Part model, mm, in its own coordinate system. Face numbers are marked on the shaded views. A direction names the side the tool comes from. Coordinates: 2 decimals unless noted, no trailing zeros. Loops run counter-clockwise (first coordinate to the right, second up) from the corner with the lowest first, then second, coordinate; pieces in that order, holes last. Notation, with made-up numbers: M -28.5,-9.75 L 15.5,-9.75 A28 ccw 15.5,29.25 Z; hole C -2.5,-7.75 d9. An arc over 180 degrees is marked long. Use a Markdown table: item, result. Add a question column.
1) Band-saw the part on C-C (z = 1.75). List the corners of the cut face in (x, y) (3 decimals).
2) Tool access for the marked faces 1, 2 and 3: list every direction of +Z, -Z, +X, -X, +Y, -Y with a clear straight run to the whole face (end or side of a thin tool).
3) Wall check: probe 1 along Y at (x, z) = (-0.5, 14.75) (3 decimals); probe 2 along Y at (x, z) = (9.75, 13.75) (3 decimals); probe 3 along Z at (x, y) = (1.75, -0.5). Give the ranges that are in metal, low to high. Write a range as from..to.
4) Pin check, flat tips, straight feed: pin 1 Ø1.5 at (x, y) = (-4, 7.5) entering from +Z; pin 2 Ø4 at (x, y) = (9.5, -2.5) entering from -Z. Stop position of each tip, or through.
5) Band-saw the part on A-A (x = 9.5). List the corners of the cut face in (y, z).
6) Band-saw the part on D-D (y = 5.5). List the corners of the cut face in (x, z).
7) Band-saw the part on B-B (y = -0.5). List the corners of the cut face in (x, z), plus the area to 3 significant figures.
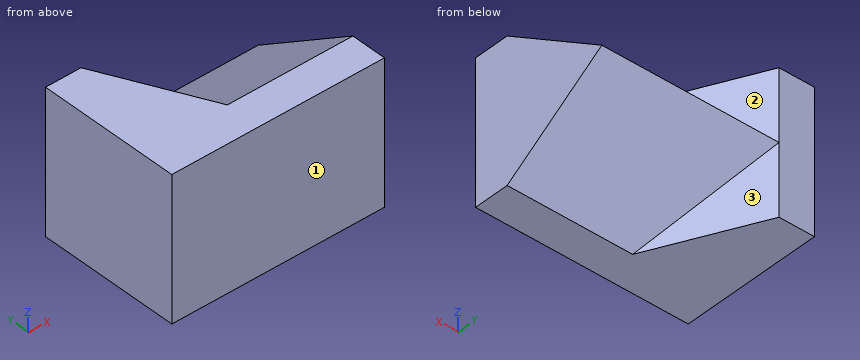
from build123d import *

# Parameters (mm, degrees)
SKETCH_1_W          = 30
SKETCH_1_H          = 20
EXTRUDE_1_DEPTH     = 20
CUT_EXTRUDE_4_DEPTH = 27.925824036
EXTRUDE_6_DEPTH     = 30


with BuildPart() as part:
    # 草圖1 → 填料-伸長1 (new body)
    with BuildSketch(Plane.XY):
        Rectangle(SKETCH_1_W, SKETCH_1_H)
    extrude(amount=EXTRUDE_1_DEPTH)

    # 草圖10 → 除料-伸長4 (cut, through all)
    with BuildSketch(Plane(origin=(0, 0, 0), x_dir=(-1, 0, 0), z_dir=(0, 0, -1))):
        Polygon((-15, -5), (2.714610503, -5), (10, 10), (-15, 10), align=None)
    extrude(amount=-CUT_EXTRUDE_4_DEPTH, mode=Mode.SUBTRACT)

    # 草圖11 → 填料-伸長6 (add)
    with BuildSketch(Plane.ZY.offset(15)):
        Polygon((0, -5), (10, 10), (20, -5), align=None)
    extrude(amount=-EXTRUDE_6_DEPTH)


solid = part.part
Entries:
| question | item | result |
|---|---|---|
| 1 | outline | M -15,-10 L 15,-10 L 15,-2.375 L -3.99,-2.375 L -10,10 L -15,10 Z |
| 2 | face 1 | +Z, -Z, +X, -X, -Y |
| 2 | face 2 | +Z, +X, +Y |
| 2 | face 3 | -Z, +X, +Y |
| 3 | probe 1 | -10..2.875 |
| 3 | probe 2 | -10..4.375 |
| 3 | probe 3 | 3..17 |
| 4 | pin 1 | z = 12.17 |
| 4 | pin 2 | z = 0.33 |
| 5 | outline | M -10,0 L -5,0 L 10,10 L -5,20 L -10,20 Z |
| 6 | outline | M -15,0 L -7.81,0 L -7.81,7 L 15,7 L 15,13 L -7.81,13 L -7.81,20 L -15,20 Z |
| 7 | outline | M -15,0 L -4.9,0 L -4.9,3 L 15,3 L 15,17 L -4.9,17 L -4.9,20 L -15,20 Z |
| 7 | area | 481 mm2 |
